Design review of the part built by this model. Coordinates are the model's own, in mm. Face numbers are marked on the shaded views. A direction names the side the tool comes from. Coordinates: 2 decimals unless noted, no trailing zeros. Loops run counter-clockwise (first coordinate to the right, second up) from the corner with the lowest first, then second, coordinate; pieces in that order, holes last. Notation, with made-up numbers: M -24.75,77 L -5.75,77 A27 cw -5.75,112 Z; hole C -31.75,17 d4. An arc over 180 degrees is marked long. Answer as a JSON object with one key per item and string values. Group by question number.
1. Consider section B-B (z = 22.75). State the section outline as (x, y) points.
2. To check wall thickness, follow probe 1 along Z at (x, y) = (-16, 21.5); probe 2 along Y at (x, z) = (27.5, 15.75); probe 3 along Y at (x, z) = (-11, 24.5). State the ranges of each line that lie inside material, in increasing order.
3. Machinability: for the marked faces 1 and 2, which of the approach directions +Z, -Z, +X, -X, +Y, -Y give a long, thin tool a straight path to every point of the face, cutting with its end or side? Answer none if there is none.
4. Insertion check: pin 1 (9.5 mm diameter, centred on x = -11, z = 11.5, fed in from -Y); pin 2 (3 mm diameter, centred on x = -5, y = -14.5, fed in from +Z). Each pin has a flat end and moves straight along its axis. Give the tip position at first contact, or say it passes through.
5. Consider section C-C (x = -15.5). State the section outline as (y, z) points.
6. Consider section A-A (y = -6.5). State the section outline as (x, z) points, then the cut area to 3 significant figures.
from build123d import *

# Parameters (mm, degrees)
F0_W     = 63.5
F0_H     = 63.5
F1_DEPTH = 25.4
F2_W     = 31.75
F2_H     = 31.75
F3_DEPTH = 19.05
F4_R     = 1.5875
F5_DEPTH = 6.35
F6_R     = 1.5875
F7_DEPTH = 38.1
F8_R     = 1.5875
F9_DEPTH = 38.1


with BuildPart() as f1:
    # F0 (on Top) → F1 (new body)
    with BuildSketch(Plane.XY):
        Rectangle(F0_W, F0_H)
    extrude(amount=F1_DEPTH)

    # F2 (on face) → F3 (cut)
    with BuildSketch(Plane.XY.offset(25.4)):
        with Locations((-15.875, -15.875)):
            Rectangle(F2_W, F2_H)
    extrude(amount=-F3_DEPTH, mode=Mode.SUBTRACT)

    # F4 (on face) → F5 (cut)
    with BuildSketch(Plane.XY.offset(6.35)):
        with Locations((-15.875, -15.875)):
            Circle(F4_R)
    extrude(amount=-F5_DEPTH, mode=Mode.SUBTRACT)

    # F6 (on face) → F7 (cut)
    with BuildSketch(Plane(origin=(0, 0, 0), x_dir=(0, -1, 0), z_dir=(-1, 0, 0))):
        with Locations((15.875, 15.875)):
            Circle(F6_R)
    extrude(amount=-F7_DEPTH, mode=Mode.SUBTRACT)

    # F8 (on face) → F9 (cut)
    with BuildSketch(Plane.XZ):
        with Locations((-15.875, 15.875576)):
            Circle(F8_R)
    extrude(amount=-F9_DEPTH, mode=Mode.SUBTRACT)


solid = f1.part
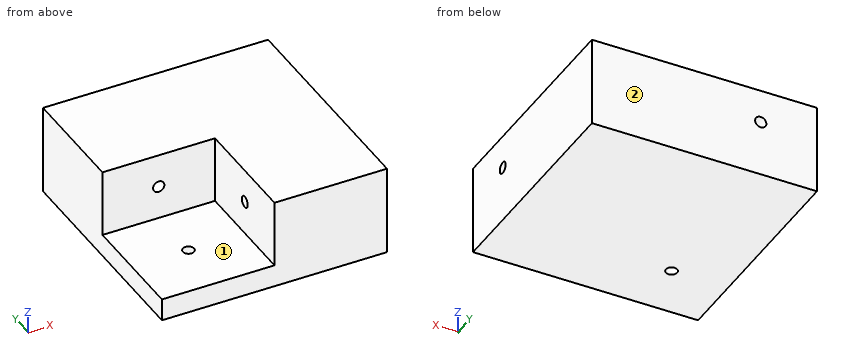
Findings below:
{
 "1": {"outline": "M -31.75,0 L 0,0 L 0,-31.75 L 31.75,-31.75 L 31.75,31.75 L -31.75,31.75 Z"},
 "2": {"probe 1": "z = 0 to 14.29, 17.46 to 25.4", "probe 2": "y = -31.75 to -17.46, -14.29 to 31.75", "probe 3": "y = 0 to 31.75"},
 "3": {"face 1": "+Z, -X, -Y", "face 2": "+Z, -Z, +X, -X, +Y"},
 "4": {"pin 1": "stops at y = 0", "pin 2": "stops at z = 6.35"},
 "5": {"outline": "M -31.75,0 L -17.42,0 L -17.42,6.35 L -31.75,6.35 Z; M -14.33,0 L 31.75,0 L 31.75,14.33 L 0,14.33 L 0,6.35 L -14.33,6.35 Z; M 0,17.42 L 31.75,17.42 L 31.75,25.4 L 0,25.4 Z"},
 "6": {"outline": "M -31.75,0 L 31.75,0 L 31.75,25.4 L 0,25.4 L 0,6.35 L -31.75,6.35 Z", "area": "1,010 mm^2"}
}
